Part model, mm, in its own coordinate system. Face numbers are marked on the shaded views. Round coordinates to 2 decimals unless told otherwise and drop trailing zeros. Loops run counter-clockwise (first coordinate to the right, second up) from the corner with the lowest first, then second, coordinate; pieces in that order, holes last.
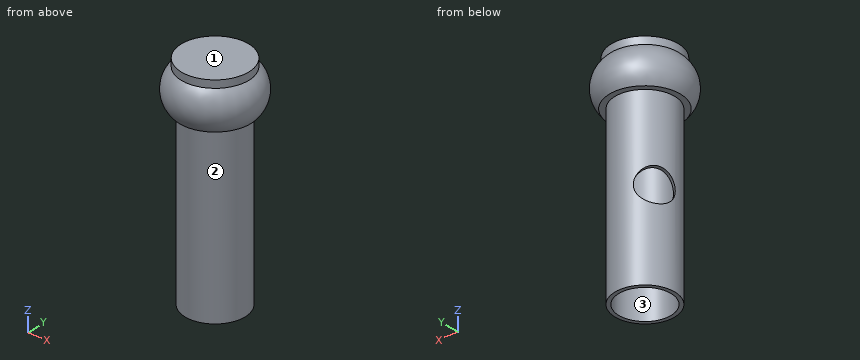
from build123d import *

# Parameters (mm, degrees)
TROU_DE_PASSAGE_D_AXE_3_321_REACH  = 43.97
TROU_DE_PASSAGE_D_AXE_3_321_BORE_R = 4.5


with BuildPart() as part:
    # Esquisse2 → Révolution1 (revolve)
    with BuildSketch(Plane(origin=(0, 0, 0), x_dir=(1, 0, 0), z_dir=(0, 1, 0)), mode=Mode.PRIVATE) as r_volution1_sk:
        with BuildLine():
            Line((7, 43.342725136), (7, -3.004612909))
            Line((7, -3.004612909), (0, -3.004612909))
            Line((0, -3.004612909), (0, -12.657274864))
            Line((0, -12.657274864), (0, -15.078606198))
            Line((0, -15.078606198), (9, -15.078606198))
            Line((9, -15.078606198), (9, -13.078606198))
            ThreePointArc((9, -13.078606198), (11.39286281, -8.14796573), (9.5, -3.004612909))
            Line((9.5, -3.004612909), (8, -3.004612909))
            Line((8, -3.004612909), (8, 43.342725136))
            Line((8, 43.342725136), (7, 43.342725136))
        make_face()
    revolve(r_volution1_sk.sketch.rotate(Axis((0, 0, -12.780225136), (0, 0, 1)), 180), axis=Axis((0, 0, -12.780225136), (0, 0, 1)))

    # Trou de passage d'axe 3/321 bore (on position points) → Trou de passage d'axe 3/321 (cut, up to next)
    with BuildSketch(Plane(origin=(-6.681517016, 4.399696622, -19.342725136), x_dir=(-0.549962077733, -0.835189627005, 0), z_dir=(-0.835189627005, 0.549962077733, 0)), mode=Mode.PRIVATE) as trou_de_passage_d_axe_3_321_sk1:
        Circle(TROU_DE_PASSAGE_D_AXE_3_321_BORE_R)
    trou_de_passage_d_axe_3_321_tool1 = extrude(trou_de_passage_d_axe_3_321_sk1.sketch, amount=-TROU_DE_PASSAGE_D_AXE_3_321_REACH, mode=Mode.PRIVATE) & part.part
    add(trou_de_passage_d_axe_3_321_tool1.solids().sort_by_distance((-6.681517, 4.399697, -19.342725))[0], mode=Mode.SUBTRACT)


solid = part.part
1) Wall check: line 1 along X through (y, z) = (0, -10); line 2 along Y through (x, z) = (-3, -29). Give the ranges that are in metal, low to high.
Values:
line 1: x = -8 to -7, 7 to 8
line 2: y = -7.42 to -6.32, 6.32 to 7.42
2) Slice it at A-A, the plane z = -8. Give the cut face in (x, y).
Values:
outline: circle Ø16 at (0, 0); hole circle Ø14 at (0, 0)
3) Drop flat-ended pins along their axis: pin 1 Ø4 at (y, z) = (1, -9) entering from +X; pin 2 Ø8 at (y, z) = (-5, -33.5) entering from +X; pin 3 Ø1.5 at (x, y) = (-7.5, -6.5) entering from +Z; pin 4 Ø4 at (x, y) = (-8, -4) entering from -Z. Give the stop position or say it passes through.
Values:
pin 1: stops at x = 8
pin 2: stops at x = 7.94
pin 3: stops at z = 12.92
pin 4: stops at z = -43.34
4) Mould opens along X. For the marked faces 1, 2 and 3 say: released by +X, released by -X, zero draft, split by the parting line, or undercut.
Values:
face 1: zero draft
face 2: split by the parting line
face 3: undercut
